```python
from build123d import *

# Parameters (mm, degrees)
EXTRUDE_1_DEPTH     = 50
SKETCH_2_R          = 1.2
CUT_EXTRUDE_1_DEPTH = 12
CHAMFER_1_SIZE      = 1.2
CHAMFER_1_SIZE2     = 0.692820323
SKETCH_3_R          = 2.1
CUT_EXTRUDE_2_DEPTH = 12
CHAMFER_2_SIZE      = 2.1
CHAMFER_2_SIZE2     = 1.212435565
CHAMFER_3_SIZE      = 0.4


with BuildPart() as part:
    # Эскиз1 → Вытянуть1 (new body)
    with BuildSketch(Plane.XY):
        Polygon((0, 4.041451884), (-3.5, 2.020725942), (-3.5, -2.020725942), (0, -4.041451884), (3.5, -2.020725942), (3.5, 2.020725942), align=None)
    extrude(amount=EXTRUDE_1_DEPTH)

    # Эскиз2 → Вырез-Вытянуть1 (cut)
    with BuildSketch(Plane.XY.offset(50)):
        Circle(SKETCH_2_R)
    extrude(amount=-CUT_EXTRUDE_1_DEPTH, mode=Mode.SUBTRACT)

    # Фаска1
    chamfer_1_edges = [part.edges().sort_by_distance(p)[0] for p in [
        (-1.2, 0, 38),
    ]]
    chamfer_1_side = [part.faces().sort_by_distance(p)[0] for p in [
        (0, 0, 38),
    ]]
    chamfer(chamfer_1_edges, length=CHAMFER_1_SIZE, length2=CHAMFER_1_SIZE2, reference=chamfer_1_side[0])

    # Эскиз3 → Вырез-Вытянуть2 (cut)
    with BuildSketch(Plane(origin=(0, 0, 0), x_dir=(-1, 0, 0), z_dir=(0, 0, -1))):
        Circle(SKETCH_3_R)
    extrude(amount=-CUT_EXTRUDE_2_DEPTH, mode=Mode.SUBTRACT)

    # Фаска2
    chamfer_2_edges = [part.edges().sort_by_distance(p)[0] for p in [
        (2.1, 0, 12),
    ]]
    chamfer_2_side = [part.faces().sort_by_distance(p)[0] for p in [
        (0, 0, 12),
    ]]
    chamfer(chamfer_2_edges, length=CHAMFER_2_SIZE, length2=CHAMFER_2_SIZE2, reference=chamfer_2_side[0])

    # Фаска3
    chamfer_3_edges = [part.edges().sort_by_distance(p)[0] for p in [
        (-1.2, 0, 50),
        (2.1, 0, 0),
    ]]
    chamfer(chamfer_3_edges, length=CHAMFER_3_SIZE)


solid = part.part
```
Input: part model. Units: mm. Frame: model coordinates. A direction names the side the tool comes from. Give positions to 0.01 mm unless a question says otherwise; leave off trailing zeros. Order: outer loops, then holes, each group sorted by start corner. A loop starts at its lowest first (then second) coordinate and runs counter-clockwise, first axis right, second up.
1. Pin query (flat end, axial travel): pin 1 Ø1.5 at (x, z) = (0.5, 39) entering from +Y; pin 2 Ø1.9 at (x, y) = (0, 0) entering from -Z. Return the tip coordinate at first contact, or that it passes through.
Computed:
pin 1: stops at y = 4.04
pin 2: stops at z = 11.45
2. Cut plane B-B (z = 41.5). Return loops of the section in (x, y).
Computed:
outline: (-3.5, -2.02) - (0, -4.04) - (3.5, -2.02) - (3.5, 2.02) - (0, 4.04) - (-3.5, 2.02) - close; hole circle Ø2.4 at (0, 0)
3. Line query: probe 1 along Y at (x, z) = (0, 47); probe 2 along Y at (x, z) = (-1.75, 9.5); probe 3 along X at (y, z) = (0.25, 4). Output: solid intervals per line, ascending.
Computed:
probe 1: y = -4.04 to -1.2, 1.2 to 4.04
probe 2: y = -3.03 to -1.16, 1.16 to 3.03
probe 3: x = -3.5 to -2.09, 2.09 to 3.5
4. Cut plane C-C (z = 13). Return loops of the section in (x, y).
Computed:
outline: (-3.5, -2.02) - (0, -4.04) - (3.5, -2.02) - (3.5, 2.02) - (0, 4.04) - (-3.5, 2.02) - close
5. Set-up query: faces 4 (the face through (0, 0, 12)), 5 (the face through (0.65, 1.01, 44.22)). Return all of +Z, -Z, +X, -X, +Y, -Y with unobstructed straight access to the full face (end or side cutting, diameter ignored); none if empty.
Computed:
face 4: -Z
face 5: +Z
6. Cut plane A-A (z = 6). Return loops of the section in (x, y).
Computed:
outline: (-3.5, -2.02) - (0, -4.04) - (3.5, -2.02) - (3.5, 2.02) - (0, 4.04) - (-3.5, 2.02) - close; hole circle Ø4.2 at (0, 0)
7. Cut plane D-D (y = -3). Return loops of the section in (x, z), and give its area (3 significant figures).
Computed:
outline: (-1.8, 0) - (1.8, 0) - (1.8, 50) - (-1.8, 50) - close
area: 180 mm2
8. Draft query along Y for faces 1 (the face through (-2.003, 0.631, 5.521)), 2 (the face through (-3.5, 0, 25)), 3 (the face through (1.726, -3.045, 24.65)). Return one class per face: released by +Y, released by -Y, zero draft, split by the parting line, or undercut.
Computed:
face 1: undercut
face 2: zero draft
face 3: released by -Y
